```python
from build123d import *

# Parameters (mm, degrees)
BOSS_EXTRUDE1_DEPTH             = 18
SKETCH2_W                       = 6
SKETCH2_H                       = 13.595638642
CUT_EXTRUDE1_DEPTH              = 10
SKETCH3_W                       = 7
SKETCH3_H                       = 13.595638642
CUT_EXTRUDE2_DEPTH              = 10
SKETCH4_R                       = 1.5
CUT_EXTRUDE3_DEPTH              = 10
TAP_DRILL_FOR_M3X0_5_TAP1_D     = 3
TAP_DRILL_FOR_M3X0_5_TAP1_DEPTH = 5
F_2_5_2_5_DIAMETER_HOLE1_D      = 2.5
F_2_5_2_5_DIAMETER_HOLE1_DEPTH  = 6.5


with BuildPart() as part:
    # Sketch1 → Boss-Extrude1 (new body)
    with BuildSketch(Plane(origin=(0, 0, 0), x_dir=(1, 0, 0), z_dir=(0, 1, 0))):
        Polygon((0, 0), (0, 6), (-7, 6), (-7, -5), (13, -5), (13, 0), align=None)
    extrude(amount=BOSS_EXTRUDE1_DEPTH)

    # Sketch2 → Cut-Extrude1 (cut)
    with BuildSketch(Plane(origin=(0, 0, 0), x_dir=(0, 0, -1), z_dir=(1, 0, 0))):
        with Locations((3, 11.202180679)):
            Rectangle(SKETCH2_W, SKETCH2_H)
    extrude(amount=-CUT_EXTRUDE1_DEPTH, mode=Mode.SUBTRACT)

    # Sketch3 → Cut-Extrude2 (cut)
    with BuildSketch(Plane(origin=(0, 0, 0), x_dir=(-1, 0, 0), z_dir=(0, 0, -1))):
        with Locations((3.5, 11.202180679)):
            Rectangle(SKETCH3_W, SKETCH3_H)
    extrude(amount=-CUT_EXTRUDE2_DEPTH, mode=Mode.SUBTRACT)

    # Sketch4 → Cut-Extrude3 (cut)
    with BuildSketch(Plane.XZ):
        with Locations((-1, -2.2)):
            Circle(SKETCH4_R)
    extrude(amount=-CUT_EXTRUDE3_DEPTH, mode=Mode.SUBTRACT)

    # Tap Drill for M3x0.5 Tap1
    with Locations(Plane(origin=(0, 0, 0), x_dir=(-1, 0, 0), z_dir=(0, -1, 0))):
        with Locations((-3.3, -2.5), (3.5, -2.5)):
            Hole(TAP_DRILL_FOR_M3X0_5_TAP1_D / 2, depth=TAP_DRILL_FOR_M3X0_5_TAP1_DEPTH)

    # Ø2.5 (2.5) Diameter Hole1
    with Locations(Plane(origin=(0, 0, 0), x_dir=(-1, 0, 0), z_dir=(0, 0, -1))):
        with Locations((-9, 14.5), (-9, 5)):
            Hole(F_2_5_2_5_DIAMETER_HOLE1_D / 2, depth=F_2_5_2_5_DIAMETER_HOLE1_DEPTH)


solid = part.part
```
Could you check a few things on this model? Use its own coordinates, in mm. A direction names the side the tool comes from. Coordinates: 2 decimals unless noted, no trailing zeros. Write each loop counter-clockwise with the first axis right and the second up, starting at its lowest first coordinate (ties: lowest second). Pieces come first, ordered by that corner, then holes. Notation, with made-up numbers: M 56.25,-32 L 76.25,-32 A7 cw 76.25,-23 Z; hole C -8.5,59 d2. An arc over 180 degrees is marked long. Answer as CSV lines item,"result". Start each with the question number.
1) Please list where these lines run through material, in increasing order: line 1 (Y direction, x = 9, z = 3.9); line 2 (Z direction, x = -2.25, y = 3.5); line 3 (Z direction, x = -3.5, y = 3.35). Write a range as from..to.
2) I want a section at C-C, the plane y = 3.5. Please give me the cut outline in (x, z), and give its area (3 significant figures).
3) I want a section at D-D, the plane x = -1.5. Please give me the cut outline in (y, z), and give its area (3 significant figures).
4) We'd pull the mould along Z, two halves only. Please class faces 5 (the cylindrical face through (3.105, 2.535, 1.013)), 6 (the flat face through (-3, 2, -6)), 7 (the flat face through (5, 9, 5)): +Z half, -Z half, draft (parallel to the pull), parting line (faces both ways), or undercut.
5) For P1, Ø5, axis at x = -3.5, z = 2.5, coming from the +Y side; P2, Ø2, axis at x = 2.5, z = -5, coming from the +Y side; P3, Ø2, axis at y = 2, z = -5, coming from the +X side; P4, Ø6.5, axis at x = 4.5, y = 12, coming from the -Z side, each with a flat end and sliding along its axis, tell me the tip position at first contact or that it passes through.
6) I want a section at B-B, the plane z = 2.5. Please give me the cut outline in (x, y), and give its area (3 significant figures).
7) For faces 1 (the flat face through (-7, 2, -1)), 2 (the flat face through (0, 11, 2)), 3 (the flat face through (0, 2, -5)), 4 (the flat face through (3, 5, 2)), which set-ups out of +Z, -Z, +X, -X, +Y, -Y let a thin tool reach every point of the face, with its end or its side?
8) I want a section at A-A, the plane y = 6. Please give me the cut outline in (x, z).
Data:
1,line 1,"y = 0..3.75, 6.25..13.25, 15.75..18"
1,line 2,"z = -6..-3.03, -1.37..1.67, 3.33..5"
1,line 3,"z = -6..1, 4..5"
2,outline,"M -7,-6 L 0,-6 L 0,-3.32 A1.5 cw long 0,-1.08 L 0,0 L 13,0 L 13,5 L -7,5 Z; hole C -3.5,2.5 d3; hole C 3.3,2.5 d3"
2,area,"122 mm^2"
3,outline,"M 0,-6 L 4.4,-6 L 4.4,-3.61 L 0,-3.61 Z; M 0,-0.79 L 4.4,-0.79 L 4.4,5 L 0,5 Z"
3,area,"36.0 mm^2"
4,face 5,"undercut"
4,face 6,"-Z half"
4,face 7,"+Z half"
5,P1,"stops at y = 4.4"
5,P2,"passes through"
5,P3,"stops at x = 0"
5,P4,"stops at z = 0"
6,outline,"M -7,0 L -5,0 L -5,4.4 L -7,4.4 Z; M -2,0 L 1.8,0 L 1.8,5 L 4.8,5 L 4.8,0 L 13,0 L 13,18 L 0,18 L 0,4.4 L -2,4.4 Z; hole C 9,5 d2.5; hole C 9,14.5 d2.5"
6,area,"227 mm^2"
7,face 1,"+Z, -Z, -X, +Y, -Y"
7,face 2,"+Z, -Z, -X, +Y"
7,face 3,"-Z, +X, +Y, -Y"
7,face 4,"-Y"
8,outline,"M 0,0 L 8.25,0 L 8.25,5 L 0,5 Z; M 9.75,0 L 13,0 L 13,5 L 9.75,5 Z"
